from build123d import *

# Parameters (mm, degrees)
SKETCH_1_R      = 35.893803705
EXTRUDE_1_DEPTH = 1.2
SHELL_1_T       = -0.5


with BuildPart() as part:
    # 스케치1 → 보스-돌출1 (new body)
    with BuildSketch(Plane(origin=(0, 0, 0), x_dir=(1, 0, 0), z_dir=(0, 1, 0))):
        with Locations(Location((0, 0, 0), (0, 0, 270))):
            Circle(SKETCH_1_R)
    extrude_1 = extrude(amount=EXTRUDE_1_DEPTH)

    # 스케치4 → 회전1 (revolve)
    with BuildSketch(Plane(origin=(0, 0, 0), x_dir=(0, 0, -1), z_dir=(1, 0, 0))):
        Polygon((-35.893803705, 1.2), (-34.159836859, 3.514461722), (-31.398977187, 4.735538278), (-30.00730795, 7.414461722), (-27.588745887, 9), (0, 9), (0, 1.2), align=None)
    revolve_1 = revolve(axis=Axis((0, 9, 0), (0, -1, 0)))

    # 대칭 복사1: 보스-돌출1, 회전1 across plane
    add(extrude_1.mirror(Plane(origin=(0, 9, 27.588745887), x_dir=(0, 0, 1), z_dir=(0, 1, 0))))
    add(revolve_1.mirror(Plane(origin=(0, 9, 27.588745887), x_dir=(0, 0, 1), z_dir=(0, 1, 0))))

    # 쉘1
    shell_1_openings = [part.faces().sort_by_distance(p)[0] for p in [
        (0, 18, 0),
        (0, 0, 0),
    ]]
    offset(amount=SHELL_1_T, openings=shell_1_openings, kind=Kind.INTERSECTION)


solid = part.part
Could you check a few things on this model? Use its own coordinates, in mm. A direction names the side the tool comes from. Give positions to 0.01 mm unless a question says otherwise; leave off trailing zeros. One line per question, with ' | ' between items. Start each with the question number.
Item 1: I'm going to push flat-ended pins straight in: pin 1 Ø1 at (y, z) = (7, -26) entering from -X; pin 2 Ø6 at (x, z) = (20, -22) entering from -Y; pin 3 Ø1 at (y, z) = (9, -16) entering from -X. Where does each tip first touch, or does it pass through?
Item 2: Thinking about a two-plate mould opening in X: for faces 1 (the cylindrical face through (10.782, 0.592, 34.236)), 2 (the conical face through (27.66, 4.29, 14.38)), 3 (the flat face through (-23.8, 18, 26.4)), which applies, pulls with the +X half, pulls with the -X half, needs draft (parallel to the pull), parting line crosses it, or undercut?
Item 3: I need wall thicknesses on probe 1 along X at (y, z) = (0.35, 0); probe 2 along X at (y, z) = (7, 12.5); probe 3 along Y at (x, z) = (11, -25.5). Which ranges of each line are inside material? Lowest first, please. Write a range as [from, to].
Item 4: For faces 4 (the cylindrical face through (35.093, 17.49, -4.608)), 5 (the conical face through (16.9, 8.9, -22)), 6 (the conical face through (-8.056, 8.906, 25.581)), which set-ups out of +Z, -Z, +X, -X, +Y, -Y let a thin tool reach every point of the face, with its end or its side?
Verdict:
1) pin 1: x = -16.36 | pin 2: y = 3.6 | pin 3: x = -23.47
2) face 1: parting line crosses it | face 2: undercut | face 3: needs draft
3) probe 1: [-35.89, -35.39], [35.39, 35.89] | probe 2: [-27.52, -26.9], [26.9, 27.52] | probe 3: [8.28, 8.88], [9.12, 9.72]
4) face 4: +Y | face 5: none | face 6: -Y
